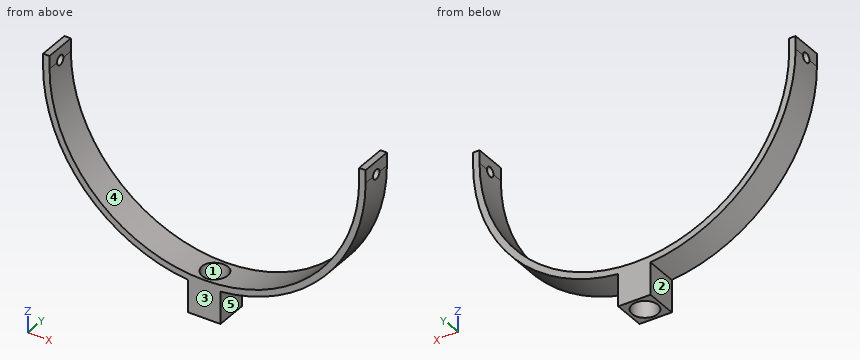
```python
from build123d import *

# Parameters (mm, degrees)
BOSS_EXTRUDE1_DEPTH = 50
SKETCH2_R           = 20
CUT_EXTRUDE1_DEPTH  = 409.166094009
SKETCH3_R           = 7.5
CUT_EXTRUDE2_DEPTH  = 585.593607558


with BuildPart() as part:
    # Sketch1 → Boss-Extrude1 (new body)
    with BuildSketch(Plane(origin=(0, 0, 0), x_dir=(1, 0, 0), z_dir=(0, 1, 0))):
        with BuildLine():
            Line((-25, 298.746859277), (25, 298.746859277))
            Line((25, 298.746859277), (25, 248.746859277))
            ThreePointArc((25, 248.746859277), (185.404962177, 167.705098312), (250, 0))
            Line((250, 0), (250, -20))
            Line((250, -20), (240, -20))
            Line((240, -20), (240, 0))
            ThreePointArc((240, 0), (0, 240), (-240, 0))
            Line((-240, 0), (-240, -20))
            Line((-240, -20), (-250, -20))
            Line((-250, -20), (-250, 0))
            ThreePointArc((-250, 0), (-185.404962177, 167.705098312), (-25, 248.746859277))
            Line((-25, 248.746859277), (-25, 298.746859277))
        make_face()
    extrude(amount=BOSS_EXTRUDE1_DEPTH)

    # Sketch2 → Cut-Extrude1 (cut, through all)
    with BuildSketch(Plane(origin=(0, 0, -298.746859277), x_dir=(-1, 0, 0), z_dir=(0, 0, -1))):
        with Locations((0, 25)):
            Circle(SKETCH2_R)
    extrude(amount=-CUT_EXTRUDE1_DEPTH, mode=Mode.SUBTRACT)

    # Sketch3 → Cut-Extrude2 (cut, through all)
    with BuildSketch(Plane.ZY.offset(250)):
        with Locations(Location((0, 25, 0), (0, 0, 90))):
            Circle(SKETCH3_R)
    extrude(amount=-CUT_EXTRUDE2_DEPTH, mode=Mode.SUBTRACT)


solid = part.part
```
Input: part model. Units: mm. Frame: model coordinates. Face numbers are marked on the shaded views. A direction names the side the tool comes from. Coordinates: 2 decimals unless noted, no trailing zeros. Loops run counter-clockwise (first coordinate to the right, second up) from the corner with the lowest first, then second, coordinate; pieces in that order, holes last. Notation, with made-up numbers: (15, 0) - (55, 0) arc R24 ccw to (55, 12) - close; hole circle Ø4 at (-30.75, 28). An arc over 180 degrees is marked (long way). Answer in a Markdown table with one row per item.
(1) Cut plane C-C on y = 25. Output: boundary loops of the cut face in (x, z).
Model answer:
| item | result |
|---|---|
| outline | (-250, 7.5) - (-240, 7.5) - (-240, 20) - (-250, 20) - close; (-249.89, -7.5) arc R250 ccw to (-25, -248.75) - (-25, -298.75) - (-20, -298.75) - (-20, -239.17) arc R240 cw to (-239.88, -7.5) - close; (20, -298.75) - (25, -298.75) - (25, -248.75) arc R250 ccw to (249.89, -7.5) - (239.88, -7.5) arc R240 cw to (20, -239.17) - close; (240, 7.5) - (250, 7.5) - (250, 20) - (240, 20) - close |
(2) Cut plane A-A on x = 0. Output: boundary loops of the cut face in (y, z), plus the area to 3 significant figures.
Model answer:
| item | result |
|---|---|
| outline | (0, -298.75) - (5, -298.75) - (5, -240) - (0, -240) - close; (45, -298.75) - (50, -298.75) - (50, -240) - (45, -240) - close |
| area | 587 mm² |
(3) Material intervals for L1, parallel to Y at x = -244, z = 0; L2, parallel to X at y = 25, z = -254; L3, parallel to Y at x = 0, z = -263, sorted ascending. Write a range as from..to.
Model answer:
| item | result |
|---|---|
| L1 | y = 0..17.5, 32.5..50 |
| L2 | x = -25..-20, 20..25 |
| L3 | y = 0..5, 45..50 |
(4) Cut plane B-B on z = -261. Output: boundary loops of the cut face in (x, y).
Model answer:
| item | result |
|---|---|
| outline | (-25, 0) - (25, 0) - (25, 50) - (-25, 50) - close; hole circle Ø40 at (0, 25) |
(5) Mould query, pull axis Y, two halves, no side actions, for the marked faces 1, 2 and 3. Classes: pulls with the +Y half, pulls with the -Y half, needs draft (parallel to the pull), parting line crosses it, or undercut.
Model answer:
| item | result |
|---|---|
| face 1 | undercut |
| face 2 | needs draft |
| face 3 | pulls with the -Y half |
(6) Pin query (flat end, axial travel): P1, Ø5, axis at y = 35, z = -230, coming from the -X side; P2, Ø3, axis at x = -12, y = 8.5, coming from the +Z side; P3, Ø10, axis at y = 22, z = -209, coming from the +X side. Return the tip coordinate at first contact, or that it passes through.
Model answer:
| item | result |
|---|---|
| P1 | stops at x = -103.65 |
| P2 | stops at z = -239.62 |
| P3 | stops at x = 144.51 |
(7) Cut plane D-D on z = -184. Output: boundary loops of the cut face in (x, y).
Model answer:
| item | result |
|---|---|
| outline | (-169.25, 0) - (-154.09, 0) - (-154.09, 50) - (-169.25, 50) - close; (154.09, 0) - (169.25, 0) - (169.25, 50) - (154.09, 50) - close |
(8) Set-up query: the marked faces 4 and 5. Return all of +Z, -Z, +X, -X, +Y, -Y with unobstructed straight access to the full face (end or side cutting, diameter ignored); none if empty.
Model answer:
| item | result |
|---|---|
| face 4 | +Z, +Y, -Y |
| face 5 | -Z, +X, +Y, -Y |
